The drawing under review shows one solid part. Ordinate dimensions are in mm from its lowest x, y, z. A direction names the side the tool comes from. Coordinates: 2 decimals unless noted, no trailing zeros. Write each loop counter-clockwise with the first axis right and the second up, starting at its lowest first coordinate (ties: lowest second). Pieces come first, ordered by that corner, then holes.
Q1. Machinability: for the marked faces 1 and 2, which of the approach directions +Z, -Z, +X, -X, +Y, -Y give a long, thin tool a straight path to every point of the face, cutting with its end or side? Answer none if there is none.
Q2. Take a section at D-D (x = 23.5). Give the boundary of the cut face in (y, z), and give its area (3 significant figures).
Q3. For probe 1 along Y at (x, z) = (12.25, 2.95); probe 2 along X at (y, z) = (13.5, 1.1); probe 3 along Y at (x, z) = (11.75, 4.85), list the stretches that pass through material, from the lowest coordinate up.
Q4. Insertion check: pin 1 (0.5 mm diameter, centred on x = 10.5, z = 3, fed in from -Y); pin 2 (2.5 mm diameter, centred on y = 3.5, z = 2, fed in from -X). Each pin has a flat end and moves straight along its axis. Give the tip position at first contact, or say it passes through.
Q5. Take a section at B-B (y = 9). Give the boundary of the cut face in (x, z), and give its area (3 significant figures).
Q6. Mouldability with a two-part tool opening along X and no side actions: class the marked faces 3, 4, 5 and 6 as pulls with the +X half, pulls with the -X half, needs draft (parallel to the pull), parting line crosses it, or undercut.
Q7. Take a section at A-A (x = 12.5). Give the boundary of the cut face in (y, z).
Q8. Take a section at C-C (z = 1.25). Give the boundary of the cut face in (x, y).
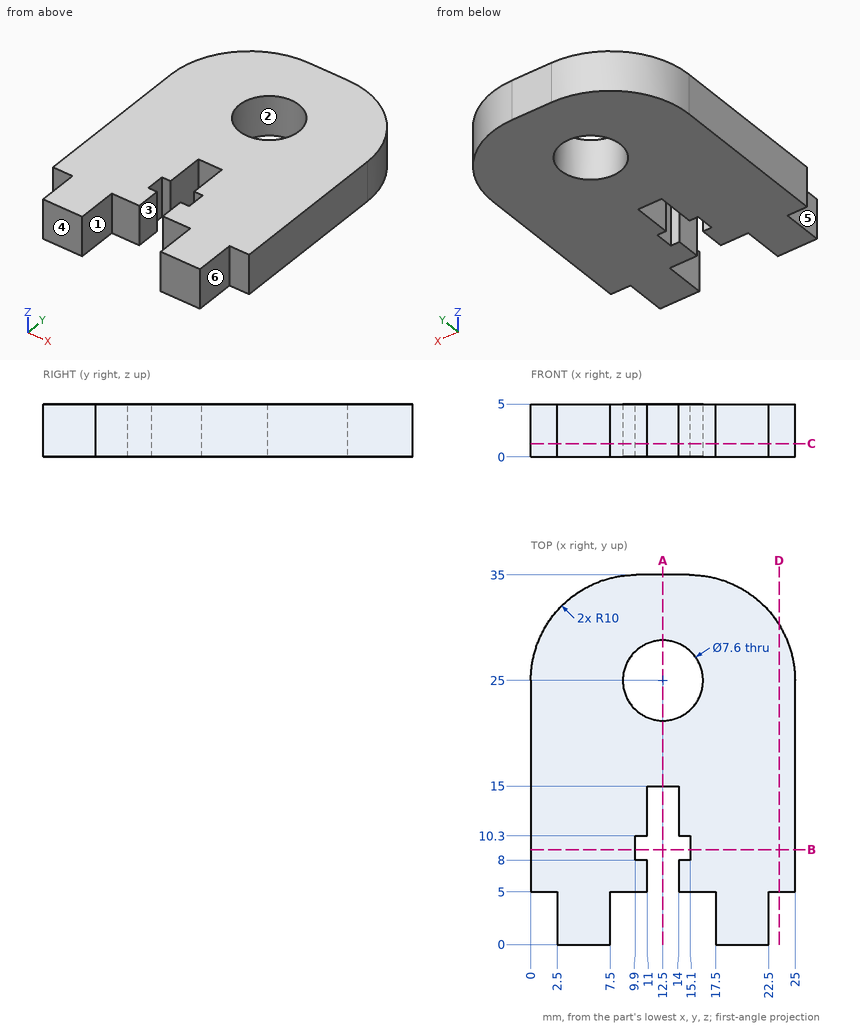
Response:
1. face 1: +Z, -Z, -Y
1. face 2: +Z, -Z
2. outline: (5, 0) - (30.27, 0) - (30.27, 5) - (5, 5) - close
2. area: 126 mm2
3. probe 1: y = 15 to 21.21, 28.79 to 35
3. probe 2: x = 0 to 11, 14 to 25
3. probe 3: y = 15 to 21.27, 28.73 to 35
4. pin 1: stops at y = 5
4. pin 2: stops at x = 2.5
5. outline: (0, 0) - (9.9, 0) - (9.9, 5) - (0, 5) - close; (15.1, 0) - (25, 0) - (25, 5) - (15.1, 5) - close
5. area: 99.0 mm2
6. face 3: undercut
6. face 4: needs draft
6. face 5: pulls with the -X half
6. face 6: pulls with the +X half
7. outline: (15, 0) - (21.2, 0) - (21.2, 5) - (15, 5) - close; (28.8, 0) - (35, 0) - (35, 5) - (28.8, 5) - close
8. outline: (0, 5) - (2.5, 5) - (2.5, 0) - (7.5, 0) - (7.5, 5) - (11, 5) - (11, 8) - (9.9, 8) - (9.9, 10.3) - (11, 10.3) - (11, 15) - (14, 15) - (14, 10.3) - (15.1, 10.3) - (15.1, 8) - (14, 8) - (14, 5) - (17.5, 5) - (17.5, 0) - (22.5, 0) - (22.5, 5) - (25, 5) - (25, 25) arc R10 ccw to (15, 35) - (10, 35) arc R10 ccw to (0, 25) - close; hole circle Ø7.6 at (12.5, 25)
